from build123d import *

# Parameters (mm, degrees)
SKETCH1_R           = 2.5
SKETCH1_W           = 5.5
SKETCH1_H           = 11
BOSS_EXTRUDE1_DEPTH = 6


with BuildPart() as part:
    # Sketch1 → Boss-Extrude1 (new body)
    with BuildSketch(Plane(origin=(0, 0, 0), x_dir=(1, 0, 0), z_dir=(0, 1, 0))):
        Polygon((0, 0), (0, 20), (42, 42.5), (62, 42.5), (108, 28), (108, 0), align=None)
        with Locations(Location((52, 30.5, 0), (0, 0, 270))):
            Circle(SKETCH1_R, mode=Mode.SUBTRACT)
        with Locations(Location((52, 10, 0), (0, 0, 270))):
            Circle(SKETCH1_R, mode=Mode.SUBTRACT)
        with Locations(Location((32, 10, 0), (0, 0, 270))):
            Circle(SKETCH1_R, mode=Mode.SUBTRACT)
        with Locations(Location((12, 10, 0), (0, 0, 270))):
            Circle(SKETCH1_R, mode=Mode.SUBTRACT)
        with Locations(Location((98, 15, 0), (0, 0, 270))):
            Circle(SKETCH1_R, mode=Mode.SUBTRACT)
        with Locations((22, 10)):
            Rectangle(SKETCH1_W, SKETCH1_H, mode=Mode.SUBTRACT)
        Polygon((40.5, 15.5), (43.5, 15.5), (44.75, 13), (44.75, 7), (43.5, 4.5), (40.5, 4.5), (39.25, 7), (39.25, 13), align=None, mode=Mode.SUBTRACT)
    extrude(amount=BOSS_EXTRUDE1_DEPTH)


solid = part.part
Part model, mm, in its own coordinate system. A direction names the side the tool comes from. Give positions to 0.01 mm unless a question says otherwise; leave off trailing zeros. Loops run counter-clockwise (first coordinate to the right, second up) from the corner with the lowest first, then second, coordinate; pieces in that order, holes last.
(1) 3-axis set-ups, long thin cutter, end or side, ignore diameter. For faces 4 (the flat face through (42, 3, -15.5)), 5 (the flat face through (55, 6, -17)): which of +Z, -Z, +X, -X, +Y, -Y reach the whole face in a straight line?
Return value:
face 4: +Y, -Y
face 5: +Z, -Z, +X, -X, +Y
(2) Band-saw the part on B-B (z = -10). Write the cut outline in (x, y).
Return value:
outline: (0, 0) - (9.5, 0) - (9.5, 6) - (0, 6) - close; (14.5, 0) - (19.25, 0) - (19.25, 6) - (14.5, 6) - close; (24.75, 0) - (29.5, 0) - (29.5, 6) - (24.75, 6) - close; (34.5, 0) - (39.25, 0) - (39.25, 6) - (34.5, 6) - close; (44.75, 0) - (49.5, 0) - (49.5, 6) - (44.75, 6) - close; (54.5, 0) - (108, 0) - (108, 6) - (54.5, 6) - close
(3) Band-saw the part on D-D (y = 2.35). Write the cut outline in (x, z), and give its area (3 significant figures).
Return value:
outline: (0, -20) - (42, -42.5) - (62, -42.5) - (108, -28) - (108, 0) - (0, 0) - close; hole circle Ø5 at (12, -10); hole (19.25, -15.5) - (24.75, -15.5) - (24.75, -4.5) - (19.25, -4.5) - close; hole circle Ø5 at (32, -10); hole (39.25, -13) - (40.5, -15.5) - (43.5, -15.5) - (44.75, -13) - (44.75, -7) - (43.5, -4.5) - (40.5, -4.5) - (39.25, -7) - close; hole circle Ø5 at (52, -30.5); hole circle Ø5 at (52, -10); hole circle Ø5 at (98, -15)
area: 3,570 mm2
(4) Band-saw the part on A-A (x = 52). Write the cut outline in (y, z).
Return value:
outline: (0, -42.5) - (6, -42.5) - (6, -33) - (0, -33) - close; (0, -28) - (6, -28) - (6, -12.5) - (0, -12.5) - close; (0, -7.5) - (6, -7.5) - (6, 0) - (0, 0) - close
(5) Band-saw the part on C-C (x = 32). Write the cut outline in (y, z), and give its area (3 significant figures).
Return value:
outline: (0, -37.14) - (6, -37.14) - (6, -12.5) - (0, -12.5) - close; (0, -7.5) - (6, -7.5) - (6, 0) - (0, 0) - close
area: 193 mm2
(6) Drill centre lines: line 1 along X through (y, z) = (2.5, -10); line 2 along X through (y, z) = (1.5, -15); line 3 along X through (y, z) = (1.85, -9). Where is each one in solid material? Low to high.
Return value:
line 1: x = 0 to 9.5, 14.5 to 19.25, 24.75 to 29.5, 34.5 to 39.25, 44.75 to 49.5, 54.5 to 108
line 2: x = 0 to 19.25, 24.75 to 40.25, 43.75 to 95.5, 100.5 to 108
line 3: x = 0 to 9.71, 14.29 to 19.25, 24.75 to 29.71, 34.29 to 39.25, 44.75 to 49.71, 54.29 to 108
(7) Pin check, flat tips, straight feed: pin 1 (6.5 mm diameter, centred on x = 98, z = -15, fed in from +Y); pin 2 (1.5 mm diameter, centred on x = 94.5, y = 0.5, fed in from -Z). Stop position of each tip, or through.
Return value:
pin 1: stops at y = 6
pin 2: stops at z = -32.49
(8) Pull direction Z, two halves, no side cores. Call faces 1 (the flat face through (55, 3, 0)), 2 (the flat face through (108, 3, -14)), 3 (the cylindrical face through (100.48, 2.96, -15.33)): pulls with the +Z half, pulls with the -Z half, needs draft (parallel to the pull), parting line crosses it, or undercut.
Return value:
face 1: pulls with the +Z half
face 2: needs draft
face 3: undercut
